```python
from build123d import *

# Parameters (mm, degrees)
SKETCH1_R           = 20
BOSS_EXTRUDE1_DEPTH = 39
SKETCH2_R           = 10
BOSS_EXTRUDE2_DEPTH = 5
SKETCH3_R           = 3
BOSS_EXTRUDE3_DEPTH = 15
FILLET1_R           = 1
SKETCH4_R           = 1.5
CUT_EXTRUDE1_DEPTH  = 5
CIRPATTERN1_COUNT   = 3


with BuildPart() as part:
    # Sketch1 → Boss-Extrude1 (new body)
    with BuildSketch(Plane.XY):
        Circle(SKETCH1_R)
    extrude(amount=BOSS_EXTRUDE1_DEPTH)

    # Sketch2 → Boss-Extrude2 (add)
    with BuildSketch(Plane.XY.offset(39)):
        Circle(SKETCH2_R)
    extrude(amount=BOSS_EXTRUDE2_DEPTH)

    # Sketch3 → Boss-Extrude3 (add)
    with BuildSketch(Plane.XY.offset(44)):
        Circle(SKETCH3_R)
    extrude(amount=BOSS_EXTRUDE3_DEPTH)

    # Fillet1
    fillet1_edges = [part.edges().sort_by_distance(p)[0] for p in [
        (-20, 0, 0),
    ]]
    fillet(fillet1_edges, radius=FILLET1_R)

    # Sketch4 → Cut-Extrude1 (cut)
    with BuildSketch(Plane.XY.offset(39)):
        with Locations((0.580678207, 14.988756213)):
            Circle(SKETCH4_R)
    cut_extrude1 = extrude(amount=-CUT_EXTRUDE1_DEPTH, mode=Mode.SUBTRACT)

    # CirPattern1: Cut-Extrude1 ×3 about axis
    cirpattern1_axis = Axis((0, 0, 0), (0, 0, 1))
    for i in range(1, CIRPATTERN1_COUNT):
        add(cut_extrude1.rotate(cirpattern1_axis, i * 360 / CIRPATTERN1_COUNT), mode=Mode.SUBTRACT)


solid = part.part
```
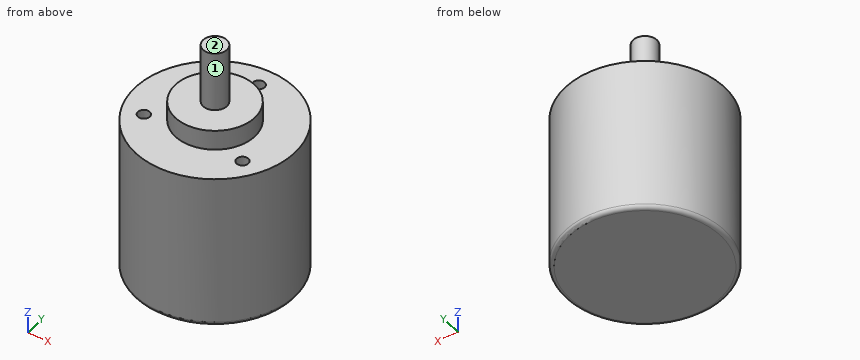
Geometry check sheet. Reference: the model listing, model coordinates, mm. Face numbers are marked on the shaded views. A direction names the side the tool comes from. Round coordinates to 2 decimals unless told otherwise and drop trailing zeros. Loops run counter-clockwise (first coordinate to the right, second up) from the corner with the lowest first, then second, coordinate; pieces in that order, holes last. Notation, with made-up numbers: (31.5, 25) -> (47.5, 25) arc R28 cw to (47.5, 60) -> close; hole circle Ø3 at (70, -29). An arc over 180 degrees is marked (long way). Use a Markdown table: item, result.
(1) Go/stop test with flat-tipped pins: P1, Ø12, axis at x = -7.5, y = -6.5, coming from the +Z side; P2, Ø2.5, axis at x = -13.5, y = -6.5, coming from the +Z side; P3, Ø0.9, axis at x = 12.5, y = -8.5, coming from the +Z side; P4, Ø12, axis at x = -10.5, y = -16, coming from the -Z side. Record where each tip stops, or that it passes through.
Calculated:
| item | result |
|---|---|
| P1 | z = 44 |
| P2 | z = 39 |
| P3 | z = 34 |
| P4 | z = 0 |
(2) Sectioned sample at D-D (z = 8). Enter the section's corners in (x, y).
Calculated:
| item | result |
|---|---|
| outline | circle Ø40 at (0, 0) |
(3) Sectioned sample at B-B (x = 0). Enter the section's corners in (y, z).
Calculated:
| item | result |
|---|---|
| outline | (-20, 1) arc R1 ccw to (-19, 0) -> (19, 0) arc R1 ccw to (20, 1) -> (20, 39) -> (16.37, 39) -> (16.37, 34) -> (13.61, 34) -> (13.61, 39) -> (10, 39) -> (10, 44) -> (3, 44) -> (3, 59) -> (-3, 59) -> (-3, 44) -> (-10, 44) -> (-10, 39) -> (-20, 39) -> close |
(4) Set-up check for the marked faces 1 and 2: record each of +Z, -Z, +X, -X, +Y, -Y from which the full face is reachable in a straight line by a thin tool's end or side.
Calculated:
| item | result |
|---|---|
| face 1 | +Z |
| face 2 | +Z, +X, -X, +Y, -Y |
(5) Sectioned sample at C-C (z = 43). Enter the section's corners in (x, y).
Calculated:
| item | result |
|---|---|
| outline | circle Ø20 at (0, 0) |
(6) Sectioned sample at A-A (y = 0). Enter the section's corners in (x, z).
Calculated:
| item | result |
|---|---|
| outline | (-20, 1) arc R1 ccw to (-19, 0) -> (19, 0) arc R1 ccw to (20, 1) -> (20, 39) -> (10, 39) -> (10, 44) -> (3, 44) -> (3, 59) -> (-3, 59) -> (-3, 44) -> (-10, 44) -> (-10, 39) -> (-20, 39) -> close |
(7) Scan lines: probe 1 along Z at (x, y) = (7, -12); probe 2 along Z at (x, y) = (5.5, 4.5); probe 3 along Y at (x, z) = (16, 24). Record each from-to range of solid material in increasing order.
Calculated:
| item | result |
|---|---|
| probe 1 | 0 to 39 |
| probe 2 | 0 to 44 |
| probe 3 | -12 to 12 |
